Source: CAD feature listing. Evaluate the final solid. Frame: model axes, mm. Round coordinates to 2 decimals unless told otherwise and drop trailing zeros. Order: outer loops, then holes, each group sorted by start corner. A loop starts at its lowest first (then second) coordinate and runs counter-clockwise, first axis right, second up. Notation, with made-up numbers: (-22, -3.5) -> (24, -3.5) arc R21 ccw to (24, 11.5) -> close; hole circle Ø3 at (-39, 88.5). An arc over 180 degrees is marked (long way). Answer as CSV lines item,"result". Start each with the question number.
(1) Section query D-D (z = 3996.5). Output: boundary loops of the cut face in (x, y).
(2) Contact query for flat-ended pins moving along their axis: P1, Ø8, axis at x = 16.5, z = 3992.5, coming from the +Y side; P2, Ø12, axis at x = 17.5, y = 181.5, coming from the +Z side; P3, Ø10, axis at x = 4, z = 3966.5, coming from the +Y side. Output: stop coordinate, or through.
(3) Section query B-B (y = 187). Count the separate pieces of the cut face and the enclosed holes in it, plus the area to 3 significant figures.
(4) Line query: line 1 along X through (y, z) = (196.5, 4011); line 2 along Z through (x, y) = (13.5, 183.25); line 3 along Z through (x, y) = (6.5, 184). Output: solid intervals per line, ascending. Write a range as from..to.
(5) Pull-direction query (Z, two-part tool) for faces 1 (the cylindrical face through (10.132, 189.373, 4015.105)), 2 (the flat face through (9.86, 191.95, 3959.166)), 3 (the flat face through (9.86, 201.823, 3989.297)), 4 (the cylindrical face through (9.86, 192.778, 3989.547)); classes: +Z half, -Z half, draft (parallel to the pull), parting line (faces both ways), or undercut.
```python
from build123d import *

# Parameters (mm, degrees)
EXTRUDE_1_DEPTH     = 20
SKETCH_3_R          = 13.5
CUT_EXTRUDE_1_DEPTH = 20
SKETCH_4_R          = 3
CUT_EXTRUDE_2_DEPTH = 22.516585743


# Read off the part's stored shape, not the designer's step: 填料-伸長1
with BuildPart() as part:
    # 填料-伸長1 outline → 填料-伸長1 (new body)
    with BuildSketch(Plane(origin=(0, 0, 0), x_dir=(0, 0, -1), z_dir=(1, 0, 0))):
        Polygon((-4019.675958787, 200.25160655), (-4018.512862627, 177.765080788), (-3958.59296353, 180.864385914), (-3959.75605969, 203.350911676), align=None)
    extrude(amount=EXTRUDE_1_DEPTH)

    # 草圖3 → 除料-伸長1 (cut)
    with BuildSketch(Plane.ZY):
        with Locations((3988.552913079, 179.314733351)):
            Circle(SKETCH_3_R)
    extrude(amount=-CUT_EXTRUDE_1_DEPTH, mode=Mode.SUBTRACT)

    # 草圖4 → 除料-伸長2 (cut)
    with BuildSketch(Plane(origin=(0, 407.076792548, 21.055696166), x_dir=(1, 0, 0), z_dir=(0, 0.9986649849421085, 0.051655085428040495))):
        with Locations(Location((10, -3950.965617011, 0), (0, 0, 270))):
            Circle(SKETCH_4_R)
    cut_extrude_2 = extrude(amount=-CUT_EXTRUDE_2_DEPTH, mode=Mode.SUBTRACT)

    # 鏡射1: 除料-伸長2 across plane
    add(cut_extrude_2.mirror(Plane(origin=(0, -205.275533435, 3968.660313072), x_dir=(1, 0, 0), z_dir=(0, 0.05165508542804326, -0.9986649849421085))), mode=Mode.SUBTRACT)


solid = part.part
```
Answer block:
1,outline,"(0, 190.23) -> (20, 190.23) -> (20, 201.45) -> (0, 201.45) -> close"
2,P1,"y = 201.86"
2,P2,"z = 4019.02"
2,P3,"y = 203.26"
3,separate pieces,"2"
3,enclosed holes,"2"
3,area,"701 mm2"
4,line 1,"0..7.39, 12.61..20"
4,line 2,"3958.72..3975.64, 4001.47..4018.8"
4,line 3,"3958.76..3975.89, 4001.21..4018.84"
5,face 1,"undercut"
5,face 2,"-Z half"
5,face 3,"+Z half"
5,face 4,"undercut"
